from build123d import *

# Parameters (mm, degrees)
F0_R     = 2.5
F1_DEPTH = 6


with BuildPart() as f1:
    # F0 (on Top) → F1 (new body)
    with BuildSketch(Plane.XY):
        Polygon((-5, 2.886751), (-5, -2.886751), (0, -5.773503), (5, -2.886751), (5, 2.886751), (0, 5.773503), align=None)
        Circle(F0_R, mode=Mode.SUBTRACT)
    extrude(amount=F1_DEPTH)

    # F2 (on Front) → F3 (revolve, intersect)
    with BuildSketch(Plane.XZ):
        Polygon((0, -2.600298), (0, 8.600298), (-9.7, 3), align=None)
    revolve(axis=Axis((0, 0, 3), (0, 0, 1)), mode=Mode.INTERSECT)


solid = f1.part
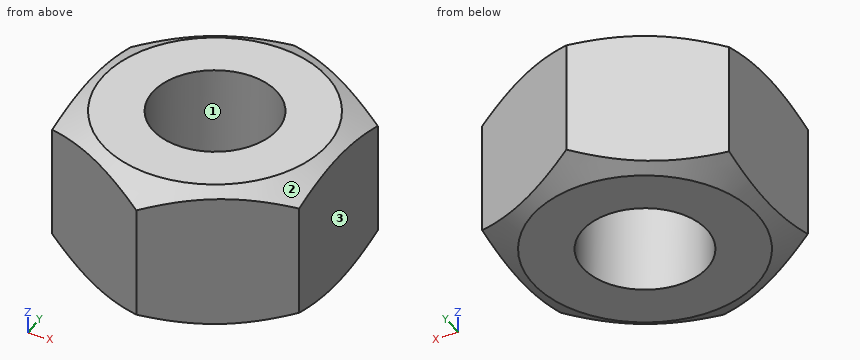
For this review, take the finished solid that the model builds, in its own axes (mm). Face numbers are marked on the shaded views. Coordinates: 2 decimals unless noted, no trailing zeros. Loops run counter-clockwise (first coordinate to the right, second up) from the corner with the lowest first, then second, coordinate; pieces in that order, holes last. Notation, with made-up numbers: (26, 27.5) -> (53, 27.5) arc R32 ccw to (53, 58.5) -> close; hole circle Ø6 at (-26, 17). An arc over 180 degrees is marked (long way). Write each question's results on one line, items separated by ' | '.
Q1. To check wall thickness, follow line 1 along Y through (x, z) = (1, 0.75); line 2 along X through (y, z) = (-1, 1.35); line 3 along Y through (x, z) = (-1.25, 1.7). State the ranges of each line that lie inside material, in increasing order. Write a range as [from, to].
Taken from the geometry:
line 1: [-5.2, -2.29], [2.29, 5.2] | line 2: [-5, -2.29], [2.29, 5] | line 3: [-5.05, -2.17], [2.17, 5.05]
Q2. Add section B-B, the plane y = 0. State the section outline as (x, z) points, then the cut area to 3 significant figures.
Taken from the geometry:
outline: (-5, 0.29) -> (-4.5, 0) -> (-2.5, 0) -> (-2.5, 6) -> (-4.5, 6) -> (-5, 5.71) -> close; (2.5, 0) -> (4.5, 0) -> (5, 0.29) -> (5, 5.71) -> (4.5, 6) -> (2.5, 6) -> close | area: 29.7 mm²
Q3. Mouldability with a two-part tool opening along Y and no side actions: class the marked faces 1, 2 and 3 as +Y half, -Y half, draft (parallel to the pull), parting line (faces both ways), or undercut.
Taken from the geometry:
face 1: undercut | face 2: parting line | face 3: draft
Q4. Add section A-A, the plane z = 2.3. State the section outline as (x, y) points, then the cut area to 3 significant figures.
Taken from the geometry:
outline: (-5, -2.89) -> (0, -5.77) -> (5, -2.89) -> (5, 2.89) -> (0, 5.77) -> (-5, 2.89) -> close; hole circle Ø5 at (0, 0) | area: 67.0 mm²
Q5. For pin 1 Ø2 at (x, z) = (1.5, 4.5) entering from +Y, flat-tipped, find the tip position at first contact; note if it passes through.
Taken from the geometry:
pin 1: y = 5.48
